Geometry: see drawing. Coordinates: mm, zero at the bounding-box minimum. Round coordinates to 2 decimals unless told otherwise and drop trailing zeros. Loops run counter-clockwise (first coordinate to the right, second up) from the corner with the lowest first, then second, coordinate; pieces in that order, holes last.
(1) Cut plane D-D, the plane y = 33.5. Output: boundary loops of the cut face in (x, z).
(2) Cut plane A-A, the plane y = 26. Output: boundary loops of the cut face in (x, z), and give its area (3 significant figures).
(3) Draft query along Y for the marked faces 1, 2 and 3. Return one class per face: released by +Y, released by -Y, zero draft, split by the parting line, or undercut.
(4) First-contact query: pin 1 Ø9 at (x, y) = (24.5, 26) entering from -Z. Flat tip, straight axial feed; report the tip coordinate or a pass-through.
(5) Line query: line 1 (Y direction, x = 5.5, z = 4); line 2 (X direction, y = 3.5, z = 12.5); line 3 (X direction, y = 24, z = 12.5). Output: solid intervals per line, ascending.
(6) Cut plane B-B, the plane x = 5.5. Output: boundary loops of the cut face in (y, z), and give its area (3 significant figures).
(7) Cut plane C-C, the plane z = 10. Output: boundary loops of the cut face in (x, y), and give its area (3 significant figures).
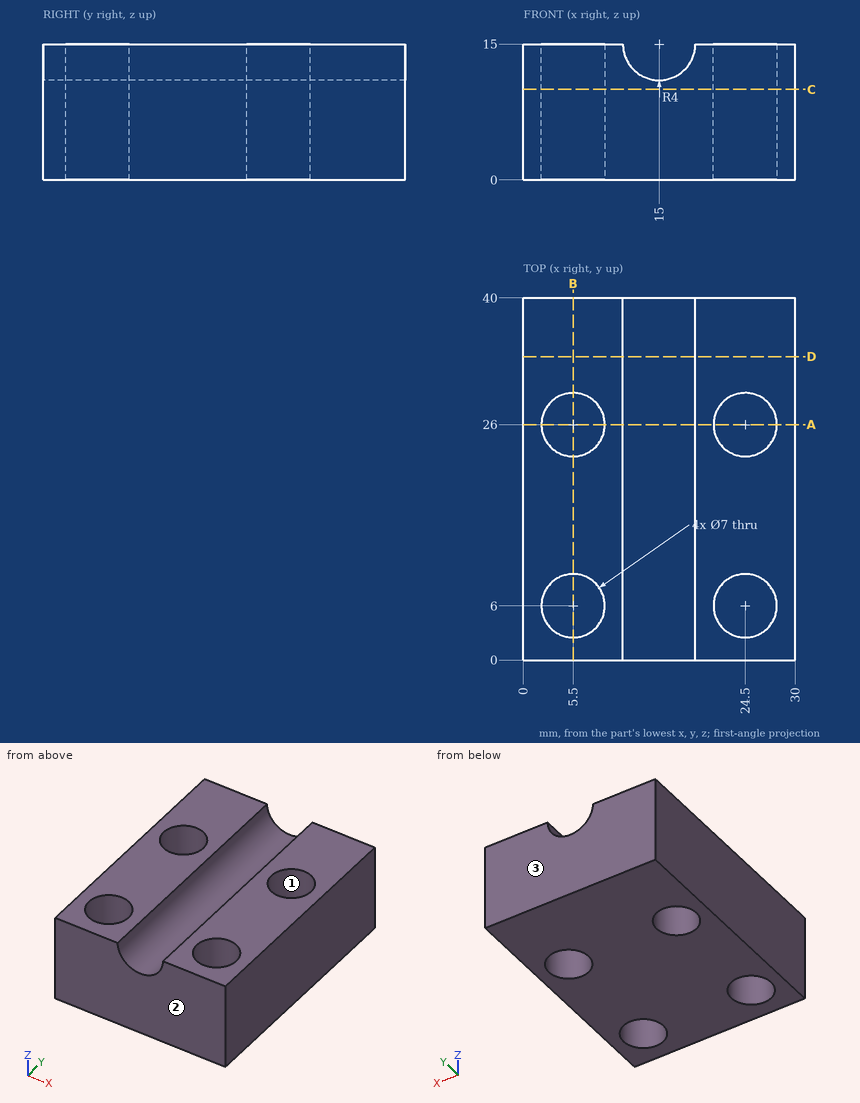
Reported:
1. outline: (0, 0) - (30, 0) - (30, 15) - (19, 15) arc R4 cw to (11, 15) - (0, 15) - close
2. outline: (0, 0) - (2, 0) - (2, 15) - (0, 15) - close; (9, 0) - (21, 0) - (21, 15) - (19, 15) arc R4 cw to (11, 15) - (9, 15) - close; (28, 0) - (30, 0) - (30, 15) - (28, 15) - close
2. area: 215 mm2
3. face 1: undercut
3. face 2: released by -Y
3. face 3: released by +Y
4. pin 1: stops at z = 0
5. line 1: y = 0 to 2.5, 9.5 to 22.5, 29.5 to 40
5. line 2: x = 0 to 3.05, 7.95 to 11.88, 18.12 to 22.05, 26.95 to 30
5. line 3: x = 0 to 2.63, 8.37 to 11.88, 18.12 to 21.63, 27.37 to 30
6. outline: (0, 0) - (2.5, 0) - (2.5, 15) - (0, 15) - close; (9.5, 0) - (22.5, 0) - (22.5, 15) - (9.5, 15) - close; (29.5, 0) - (40, 0) - (40, 15) - (29.5, 15) - close
6. area: 390 mm2
7. outline: (0, 0) - (30, 0) - (30, 40) - (0, 40) - close; hole circle Ø7 at (5.5, 6); hole circle Ø7 at (5.5, 26); hole circle Ø7 at (24.5, 6); hole circle Ø7 at (24.5, 26)
7. area: 1,050 mm2
